Design review of the part built by this model. Coordinates are the model's own, in mm. Give positions to 0.01 mm unless a question says otherwise; leave off trailing zeros. Loops run counter-clockwise (first coordinate to the right, second up) from the corner with the lowest first, then second, coordinate; pieces in that order, holes last. Notation, with made-up numbers: (36, 77) -> (42, 77) arc R15 ccw to (42, 85) -> close; hole circle Ø2 at (-26.5, 20.25). An arc over 180 degrees is marked (long way). Answer as CSV lines item,"result".
from build123d import *

# Parameters (mm, degrees)
BOSS_EXTRU_1_DEPTH = 5


with BuildPart() as part:
    # Esquisse1 → Boss.-Extru.1 (new body)
    with BuildSketch(Plane.XY):
        with BuildLine():
            Line((0, 0), (-15.5, 0))
            Line((-15.5, 0), (-15.5, -25.5))
            Line((-15.5, -25.5), (-20.5, -25.5))
            Line((-20.5, -25.5), (-20.5, -35.5))
            Line((-20.5, -35.5), (-15.5, -35.5))
            Line((-15.5, -35.5), (-15.5, -54.5))
            Line((-15.5, -54.5), (180.5, -54.5))
            Line((180.5, -54.5), (180.5, -35.5))
            Line((180.5, -35.5), (185.5, -35.5))
            Line((185.5, -35.5), (185.5, -25.5))
            Line((185.5, -25.5), (180.5, -25.5))
            Line((180.5, -25.5), (180.5, 0))
            Line((180.5, 0), (165, 0))
            ThreePointArc((165, 0), (82.5, -45), (0, 0))
        make_face()
    extrude(amount=BOSS_EXTRU_1_DEPTH)


solid = part.part
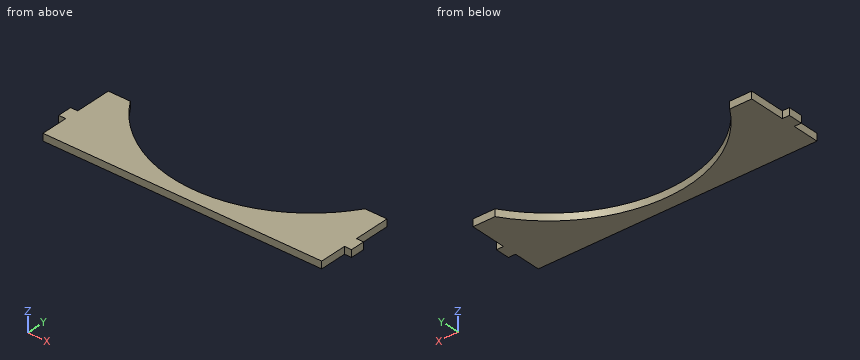
Q1. We need section B-B, the plane z = 0.8. State the section outline as (x, y) points (3 decimals), and give its area (3 significant figures).
Filled sheet:
outline,"(-20.5, -35.5) -> (-15.5, -35.5) -> (-15.5, -54.5) -> (180.5, -54.5) -> (180.5, -35.5) -> (185.5, -35.5) -> (185.5, -25.5) -> (180.5, -25.5) -> (180.5, 0) -> (165, 0) arc R98.125 cw to (0, 0) -> (-15.5, 0) -> (-15.5, -25.5) -> (-20.5, -25.5) -> close"
area,"5,550 mm^2"
Q2. Clearance check with flat-ended pins moving along their axes: pin 1 Ø1.5 at (x, z) = (-17, 3.5) entering from +Y; pin 2 Ø1.5 at (x, z) = (182.5, 3.5) entering from -Y; pin 3 Ø1.5 at (y, z) = (-40.5, 2) entering from -X; pin 4 Ø1 at (x, y) = (93.5, -42.5) entering from +Z. State where each tip first meets the part, or that it passes through.
Filled sheet:
pin 1,"stops at y = -25.5"
pin 2,"stops at y = -35.5"
pin 3,"stops at x = -15.5"
pin 4,"passes through"
Q3. We need section A-A, the plane y = -29. State the section outline as (x, z) points.
Filled sheet:
outline,"(-20.5, 0) -> (28.8, 0) -> (28.8, 5) -> (-20.5, 5) -> close; (136.2, 0) -> (185.5, 0) -> (185.5, 5) -> (136.2, 5) -> close"
Q4. We need section D-D, the plane x = 148. State the section outline as (y, z) points.
Filled sheet:
outline,"(-54.5, 0) -> (-19.94, 0) -> (-19.94, 5) -> (-54.5, 5) -> close"
Q5. We need section C-C, the plane y = -16. State the section outline as (x, z) points.
Filled sheet:
outline,"(-15.5, 0) -> (12.86, 0) -> (12.86, 5) -> (-15.5, 5) -> close; (152.14, 0) -> (180.5, 0) -> (180.5, 5) -> (152.14, 5) -> close"
Q6. To check wall thickness, follow probe 1 along X at (y, z) = (-49.5, 1.75); probe 2 along X at (y, z) = (-29.5, 4.4); probe 3 along Y at (x, z) = (81, 1.25). State the ranges of each line that lie inside material, in increasing order. Write a range as from..to.
Filled sheet:
probe 1,"x = -15.5..180.5"
probe 2,"x = -20.5..29.57, 135.43..185.5"
probe 3,"y = -54.5..-44.99"
